from build123d import *

# Parameters (mm, degrees)
SKETCH_1_W          = 129.5
SKETCH_1_H          = 189.5
EXTRUDE_1_DEPTH     = 1
SKETCH_2_W          = 115.8
SKETCH_2_H          = 174.8
SKETCH_2_W_2        = 111.8
SKETCH_2_H_2        = 170.8
EXTRUDE_2_DEPTH     = 1.5
SKETCH_3_W          = 7.9
SKETCH_3_H          = 30
CUT_EXTRUDE_1_DEPTH = 3


with BuildPart() as part:
    # 草图1 → 凸台-拉伸1 (new body)
    with BuildSketch(Plane.XY):
        Rectangle(SKETCH_1_W, SKETCH_1_H)
    extrude(amount=EXTRUDE_1_DEPTH)

    # 草图2 → 凸台-拉伸2 (add)
    with BuildSketch(Plane.XY.offset(1)):
        with Locations((2.9, 0)):
            Rectangle(SKETCH_2_W, SKETCH_2_H)
        with Locations((2.9, 0)):
            Rectangle(SKETCH_2_W_2, SKETCH_2_H_2, mode=Mode.SUBTRACT)
    extrude(amount=EXTRUDE_2_DEPTH)

    # 草图3 → 切除-拉伸1 (cut)
    with BuildSketch(Plane.XY.offset(2.5)):
        with Locations((60.8, 0)):
            Rectangle(SKETCH_3_W, SKETCH_3_H)
    extrude(amount=-CUT_EXTRUDE_1_DEPTH, mode=Mode.SUBTRACT)


solid = part.part
Model file for the job. Use its own axes, mm. Give positions to 0.01 mm unless a question says otherwise; leave off trailing zeros. Loops run counter-clockwise (first coordinate to the right, second up) from the corner with the lowest first, then second, coordinate; pieces in that order, holes last.
1) Pull direction Y, two halves, no side cores. Call faces 1 (the flat face through (-1, 1, 0)), 2 (the flat face through (2, 1, 1)): +Y half, -Y half, draft (parallel to the pull), parting line (faces both ways), or undercut.
2) Saw through at A-A (z = 1.85). Write the cut outline in (x, y).
3) Saw through at B-B (x = -13). Write the cut outline in (y, z), plus the area to 4 significant figures.
4) Wall check: line 1 (X direction, y = 29, z = 1.7); line 2 (Y direction, x = -41, z = 1.75); line 3 (Z direction, x = 24, y = -70.5). Give the ranges that are in metal, low to high.
5) Flat gauge pins, fed straight in: pin 1 Ø0.8 at (y, z) = (-61, 2) entering from -X; pin 2 Ø1.2 at (y, z) = (63.5, 2) entering from +X; pin 3 Ø1.2 at (y, z) = (-5.5, 2) entering from +X. Where does each tip first touch, or does it go through?
Answer block:
1. face 1: draft
1. face 2: undercut
2. outline: (-55, -87.4) - (60.8, -87.4) - (60.8, -15) - (58.8, -15) - (58.8, -85.4) - (-53, -85.4) - (-53, 85.4) - (58.8, 85.4) - (58.8, 15) - (60.8, 15) - (60.8, 87.4) - (-55, 87.4) - close
3. outline: (-94.75, 0) - (94.75, 0) - (94.75, 1) - (87.4, 1) - (87.4, 2.5) - (85.4, 2.5) - (85.4, 1) - (-85.4, 1) - (-85.4, 2.5) - (-87.4, 2.5) - (-87.4, 1) - (-94.75, 1) - close
3. area: 195.5 mm2
4. line 1: x = -55 to -53, 58.8 to 60.8
4. line 2: y = -87.4 to -85.4, 85.4 to 87.4
4. line 3: z = 0 to 1
5. pin 1: stops at x = -55
5. pin 2: stops at x = 60.8
5. pin 3: stops at x = -53
